Geometry check sheet. Reference: the model listing, model coordinates, mm. Face numbers are marked on the shaded views. A direction names the side the tool comes from. Round coordinates to 2 decimals unless told otherwise and drop trailing zeros. Write each loop counter-clockwise with the first axis right and the second up, starting at its lowest first coordinate (ties: lowest second). Pieces come first, ordered by that corner, then holes. Notation, with made-up numbers: (-31, 57) -> (11, 57) arc R27 cw to (11, 84) -> close; hole circle Ø10 at (13, -33). An arc over 180 degrees is marked (long way). Use a Markdown table: item, result.
```python
from build123d import *

# Parameters (mm, degrees)
BOSS_EXTRUDE1_DEPTH      = 30
BOSS_EXTRUDE1_DEPTH_BACK = 30
SKETCH2_R                = 3.25
SKETCH2_R_2              = 1.25
SKETCH2_R_3              = 5
SKETCH3_W                = 58
SKETCH3_H                = 55
CUT_EXTRUDE1_DEPTH       = 60.373815778
SKETCH4_W                = 10
SKETCH4_H                = 8
BOSS_EXTRUDE2_DEPTH      = 10
FILLET1_R                = 4
SKETCH5_R                = 1.75
CUT_EXTRUDE2_DEPTH       = 76.599272483
FILLET1_OF_MIRROR1_R     = 4
FILLET2_R                = 4
SKETCH6_R                = 1.25
SKETCH6_R_2              = 5
BOSS_EXTRUDE3_DEPTH      = 3
SKETCH7_R                = 2.5
CUT_EXTRUDE3_DEPTH       = 2


with BuildPart() as part:
    # Sketch2 → Boss-Extrude1 (new, two sides: drawn at the far end of the back side and taken through both)
    with BuildSketch(Plane.XY.offset(-BOSS_EXTRUDE1_DEPTH_BACK)):
        with BuildLine():
            Line((-7.5, 5), (-7.5, 30))
            Line((-7.5, 30), (5.086494468, 45))
            Line((5.086494468, 45), (24.5, 45))
            Line((24.5, 45), (24.5, 20))
            Line((24.5, 20), (7.5, 20))
            Line((7.5, 20), (7.5, 5))
            ThreePointArc((7.5, 5), (6.035533906, 1.464466094), (2.5, 0))
            Line((2.5, 0), (-2.5, 0))
            ThreePointArc((-2.5, 0), (-6.035533906, 1.464466094), (-7.5, 5))
        make_face()
        with Locations((0, 5)):
            Circle(SKETCH2_R, mode=Mode.SUBTRACT)
        with Locations((18.004770913, 32.569673822)):
            Circle(SKETCH2_R_2, mode=Mode.SUBTRACT)
        with Locations((-0.995229087, 32.569673822)):
            Circle(SKETCH2_R_2, mode=Mode.SUBTRACT)
        with Locations((8.504770913, 29.569673822)):
            Circle(SKETCH2_R_3, mode=Mode.SUBTRACT)
    extrude(amount=BOSS_EXTRUDE1_DEPTH + BOSS_EXTRUDE1_DEPTH_BACK)

    # Sketch3 → Cut-Extrude1 (cut, through all)
    with BuildSketch(Plane(origin=(0, 45, 0), x_dir=(1, 0, 0), z_dir=(0, 1, 0))):
        with Locations((-7.5, 0)):
            Rectangle(SKETCH3_W, SKETCH3_H)
    extrude(amount=-CUT_EXTRUDE1_DEPTH, mode=Mode.SUBTRACT)

    # Sketch4 → Boss-Extrude2 (add)
    with BuildSketch(Plane(origin=(24.5, 0, 0), x_dir=(0, 0, -1), z_dir=(1, 0, 0))):
        with Locations((-25, 41)):
            Rectangle(SKETCH4_W, SKETCH4_H)
    boss_extrude2 = extrude(amount=BOSS_EXTRUDE2_DEPTH)

    # Fillet1
    fillet1_edges = [part.edges().sort_by_distance(p)[0] for p in [
        (34.5, 37, 25),
        (34.5, 45, 25),
    ]]
    fillet(fillet1_edges, radius=FILLET1_R - 0.0001)  # a hair under: the kernel refuses the full size

    # Sketch5 → Cut-Extrude2 (cut, through all)
    with BuildSketch(Plane(origin=(0, 0, 20), x_dir=(-1, 0, 0), z_dir=(0, 0, -1))):
        with Locations((-30.5, 41)):
            Circle(SKETCH5_R)
    cut_extrude2 = extrude(amount=-CUT_EXTRUDE2_DEPTH, mode=Mode.SUBTRACT)

    # Mirror1: Boss-Extrude2, Cut-Extrude2 across plane
    add(boss_extrude2.mirror(Plane.XY))
    add(cut_extrude2.mirror(Plane.XY), mode=Mode.SUBTRACT)

    # Fillet1 of Mirror1
    fillet1_of_mirror1_edges = [part.edges().sort_by_distance(p)[0] for p in [
        (34.5, 37, -25),
        (34.5, 45, -25),
    ]]
    fillet(fillet1_of_mirror1_edges, radius=FILLET1_OF_MIRROR1_R - 0.0001)  # a hair under: the kernel refuses the full size

    # Fillet2
    fillet2_edges = [part.edges().sort_by_distance(p)[0] for p in [
        (24.5, 37, 25),
        (24.5, 41, 20),
        (24.5, 37, -25),
        (24.5, 41, -20),
        (5.086494468, 45, -28.75),
        (7.5, 20, -28.75),
        (-7.5, 30, -28.75),
        (-7.5, 30, 28.75),
        (7.5, 20, 28.75),
        (5.086494468, 45, 28.75),
    ]]
    fillet(fillet2_edges, radius=FILLET2_R)

    # Sketch6 → Boss-Extrude3 (add)
    with BuildSketch(Plane.XY.offset(-27.5)):
        with BuildLine():
            Line((21.5, 45), (6.9517251, 45))
            ThreePointArc((6.9517251, 45), (5.261252053, 44.625231148), (3.887547328, 43.571150439))
            Line((3.887547328, 43.571150439), (-6.564177772, 31.115269502))
            ThreePointArc((-6.564177772, 31.115269502), (-7.258770483, 29.912199636), (-7.5, 28.544119063))
            ThreePointArc((-7.5, 28.544119063), (0.776489044, 21.551274863), (11.5, 20))
            Line((11.5, 20), (21.5, 20))
            Line((21.5, 20), (21.5, 45))
        make_face()
        with Locations((18.004770913, 32.569673822)):
            Circle(SKETCH6_R, mode=Mode.SUBTRACT)
        with Locations((8.504770913, 29.569673822)):
            Circle(SKETCH6_R_2, mode=Mode.SUBTRACT)
        with Locations((-0.995229087, 32.569673822)):
            Circle(SKETCH6_R, mode=Mode.SUBTRACT)
    boss_extrude3 = extrude(amount=BOSS_EXTRUDE3_DEPTH)

    # Sketch7 → Cut-Extrude3 (cut)
    with BuildSketch(Plane(origin=(0, 0, -30), x_dir=(-1, 0, 0), z_dir=(0, 0, -1))):
        with Locations((-18.004770913, 32.569673822)):
            Circle(SKETCH7_R)
        with Locations((0.995229087, 32.569673822)):
            Circle(SKETCH7_R)
    cut_extrude3 = extrude(amount=-CUT_EXTRUDE3_DEPTH, mode=Mode.SUBTRACT)

    # Mirror2: Boss-Extrude3, Cut-Extrude3 across plane
    add(boss_extrude3.mirror(Plane.XY))
    add(cut_extrude3.mirror(Plane.XY), mode=Mode.SUBTRACT)


solid = part.part
```
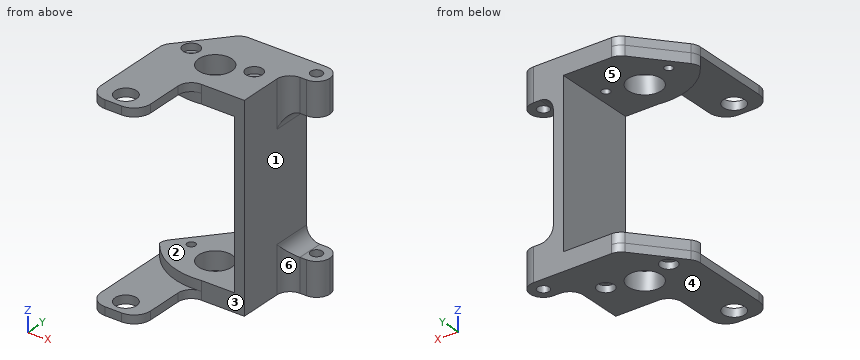
(1) Thickness scan on line 1 (Z direction, x = -4, y = 12); line 2 (X direction, y = 5, z = -29.3); line 3 (Z direction, x = 18.5, y = 42). Record the ranges inside material, lowest first.
A:
| item | result |
|---|---|
| line 1 | z = -30 to -27.5, 27.5 to 30 |
| line 2 | x = -7.5 to -3.25, 3.25 to 7.5 |
| line 3 | z = -30 to -24.5, 24.5 to 30 |
(2) Access from +Z, -Z, +X, -X, +Y, -Y to the whole of each face (thin tool, end or side, straight path). Record for the marked faces 1, 2 and 3.
A:
| item | result |
|---|---|
| face 1 | +X, -Y |
| face 2 | -X, +Y, -Y |
| face 3 | +Z, -Z, +X, -Y |
(3) Section check A-A on y = 11.5. Record the cut outline in (x, z).
A:
| item | result |
|---|---|
| outline | (-7.5, -30) -> (7.5, -30) -> (7.5, -27.5) -> (-7.5, -27.5) -> close; (-7.5, 27.5) -> (7.5, 27.5) -> (7.5, 30) -> (-7.5, 30) -> close |
(4) Section check B-B on z = 8.5. Record the cut outline in (x, y).
A:
| item | result |
|---|---|
| outline | (21.5, 20) -> (24.5, 20) -> (24.5, 45) -> (21.5, 45) -> close |
(5) Release check for a two-part mould opening along Z. For the marked faces 4, 5 and 6 record: +Z half, -Z half, draft (parallel to the pull), parting line (faces both ways), or undercut.
A:
| item | result |
|---|---|
| face 4 | -Z half |
| face 5 | undercut |
| face 6 | draft |
(6) Gauge pin test, flat ends, axial feed: pin 1 Ø1 at (y, z) = (29, -17.5) entering from -X; pin 2 Ø1.6 at (x, z) = (29, -24.5) entering from -Y; pin 3 Ø3 at (x, y) = (-1, 32.57) entering from -Z. Record the tip position at first contact, or that the pin passes through.
A:
| item | result |
|---|---|
| pin 1 | stops at x = 21.5 |
| pin 2 | stops at y = 36.99 |
| pin 3 | stops at z = -28 |
